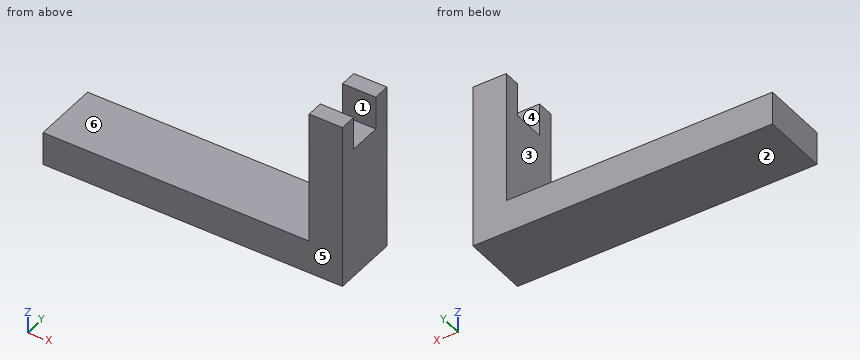
```python
from build123d import *

# Parameters (mm, degrees)
BOX_W     = 20
BOX_H     = 10
BOX_DEPTH = 10
PAD_DEPTH = 20


with BuildPart() as cubo:
    # Box → Box (new body)
    with BuildSketch(Plane(origin=(76, 5, 40), x_dir=(1, 0, 0), z_dir=(0, 0, 1))):
        with Locations((10, 5)):
            Rectangle(BOX_W, BOX_H)
    extrude(amount=BOX_DEPTH)


with BuildPart() as cut001:
    # Sketch → Pad (new body)
    with BuildSketch(Plane.XZ):
        Polygon((0, 0), (90, 0), (90, 50), (80, 50), (80, 10), (0, 10), align=None)
    extrude(amount=PAD_DEPTH)


with BuildPart() as cut001_1:
    # Body placement: moved
    add(cut001.part.moved(Location((0, 20, 0))))

    # Cut001: cut Cubo
    add(cubo.part, mode=Mode.SUBTRACT)


solid = cut001_1.part
```
Here's how the part is built. I have some questions about the finished solid (model axes, mm). Face numbers are marked on the shaded views. A direction names the side the tool comes from. Coordinates: 2 decimals unless noted, no trailing zeros. Order: outer loops, then holes, each group sorted by start corner. A loop starts at its lowest first (then second) coordinate and runs counter-clockwise, first axis right, second up. Notation, with made-up numbers: M 54.5,60 L 106.5,60 A32 cw 106.5,90 Z; hole C 9.5,24 d1. An arc over 180 degrees is marked long. Answer as a JSON object with one key per item and string values. Group by question number.
(1) For pin 1 (6 mm diameter, centred on x = 40, y = 11.5, fed in from +Z); pin 2 (8 mm diameter, centred on x = 84, y = 8.5, fed in from +Z); pin 3 (1.5 mm diameter, centred on y = 5.5, z = 26, fed in from -X), each with a flat end and sliding along its axis, tell me the tip position at first contact or that it passes through.
(2) Suppose I cut it at A-A, the plane z = 46.5. Please give me the cut outline in (x, y).
(3) Suppose I cut it at C-C, the plane x = 60. Please give me the cut outline in (y, z).
(4) Suppose I cut it at D-D, the plane z = 24. Please give me the cut outline in (x, y), then the cut area to 3 significant figures.
(5) Suppose I cut it at B-B, the plane y = 9.75. Please give me the cut outline in (x, z), then the cut area to 3 significant figures.
(6) If we mould it in two halves opening along Y, with no side actions, what happens to the marked faces 4, 5 and 6? For each: released by +Y, released by -Y, zero draft, split by the parting line, or undercut.
(7) Which directions (+Z, -Z, +X, -X, +Y, -Y) give clear straight access to the entire face, cutting with the end or side of a thin tool? Please do the marked faces 1, 2 and 3.
(8) I need wall thicknesses on probe 1 along X at (y, z) = (1, 35); probe 2 along Z at (x, y) = (75, 1.5). Which ranges of each line are inside material? Lowest first, please.
Values found:
{
 "1": {"pin 1": "stops at z = 10", "pin 2": "stops at z = 50", "pin 3": "stops at x = 80"},
 "2": {"outline": "M 80,0 L 90,0 L 90,5 L 80,5 Z; M 80,15 L 90,15 L 90,20 L 80,20 Z"},
 "3": {"outline": "M 0,0 L 20,0 L 20,10 L 0,10 Z"},
 "4": {"outline": "M 80,0 L 90,0 L 90,20 L 80,20 Z", "area": "200 mm^2"},
 "5": {"outline": "M 0,0 L 90,0 L 90,40 L 80,40 L 80,10 L 0,10 Z", "area": "1,200 mm^2"},
 "6": {"face 4": "undercut", "face 5": "released by -Y", "face 6": "zero draft"},
 "7": {"face 1": "+Z, +X, -X", "face 2": "-Z, +X, -X, +Y, -Y", "face 3": "+Z, -X, +Y, -Y"},
 "8": {"probe 1": "x = 80 to 90", "probe 2": "z = 0 to 10"}
}
